Autodesk Inventor part; units mm, degrees
ref_plane "YZ Plane" through (0, 0, 0) normal (1, 0, 0) x (0, 1, 0)
ref_plane "XZ Plane" through (0, 0, 0) normal (0, 1, 0) x (-1, 0, 0)
ref_plane "XY Plane" through (0, 0, 0) normal (0, 0, 1) x (1, 0, 0)
sketch "Sketch3" plane through (0, 0, 0) normal (0, 1, 0) x (-1, 0, 0)
  line L0 (0, 0) -> (10, 0)
  line L1 (10, 0) -> (10, -10)
  line L2 (10, -10) -> (0, -10)
  line L3 (0, -10) -> (0, 0)
  dimension "d7" = 10
  dimension "d8" = 10
extrude "Extrusion1" add sketch "Sketch3" along normal blind 10
sketch "Sketch4" plane through (0, 0, 0) normal (1, 0, 0) x (0, 0, -1)
  line L0 (10, 0) -> (0, 0)
  line L1 (0, 0) -> (0, 10)
  line L2 (0, 0) -> (2.5, 0)
  line L3 (2.5, 0) -> (0, 2.3259)
  dimension "d11" = 2.5
extrude "Extrusion2" cut sketch "Sketch4" against normal blind 10
sketch "Sketch5" plane through (0, 0, -10) normal (1, 0, 0) x (0, 0, -1)
  line L0 (0, 0) -> (-7.5, 0)
  line L1 (0, 0) -> (0, 10)
  line L2 (-10, 10) -> (0, 10)
  line L3 (-10, 2.3259) -> (-10, 10)
  line L4 (-3.75, 0) -> (-3.75, 2.3259)
  line L5 (-3.75, 2.3259) -> (0, 4.4117)
  line L6 (0, 0) -> (-3.75, 0)
  line L7 (-1.5, 10) -> (-1.5, 6)
  line L8 (-1.5, 6) -> (-4.6791, 10)
  point P0 (-10, 0)
  dimension "d14" = 4
extrude "Extrusion3" cut sketch "Sketch5" against normal blind 10 contours L0 L4 L5 L1
sketch "Sketch6" plane through (0, 10, 0) normal (1, 0, 0) x (0, 0, -1)
  line L0 (0, 0) -> (10, 0)
  line L1 (6.25, -10) -> (2.5, -10)
  line L2 (8.75, 0) -> (8.75, -4.6256)
  line L3 (8.75, -4.6256) -> (5, 0)
  line L4 (5, 0) -> (8.75, 0)
  point P0 (0, -10)
extrude "Extrusion4" cut sketch "Sketch6" against normal blind 10
sketch "Sketch7" plane through (0, 2.3259, 0) normal (1, 0, 0) x (0, 0, -1)
  line L0 (0, 7.6741) -> (5, 7.6741)
  line L1 (0, 0) -> (0, 7.6741)
  line L2 (3.0747, 7.6741) -> (0, 7.6741)
  line L3 (0, 7.6741) -> (0, 2.0858)
  line L4 (0, 2.0858) -> (3.0747, 2.0858)
  line L5 (3.0747, 2.0858) -> (3.0747, 7.6741)
  point P0 (0, -2.3259)
extrude "Extrusion5" cut sketch "Sketch7" against normal blind 10
properties part number "136"
Build history of the part. All positions in model axes, mm. A direction names the side the tool comes from. Round coordinates to 2 decimals unless told otherwise and drop trailing zeros. Write each loop counter-clockwise with the first axis right and the second up, starting at its lowest first coordinate (ties: lowest second). Pieces come first, ordered by that corner, then holes.
1) Drill centre lines: probe 1 along Z at (x, y) = (-3, 7); probe 2 along Z at (x, y) = (-8.5, 9.25); probe 3 along Z at (x, y) = (-6.25, 4). Where is each one in solid material? Low to high.
2) 3-axis set-ups, long thin cutter, end or side, ignore diameter. For faces 1 (the flat face through (-5, 10, -4)), 2 (the flat face through (-5, 1, -6.25)), 3 (the flat face through (-5, 7, -3.075)): which of +Z, -Z, +X, -X, +Y, -Y reach the whole face in a straight line?
3) Mould opens along Z. For faces 4 (the flat face through (-5, 8, -8.75)), 5 (the flat face through (-5, 4.412, -2)), 6 (the flat face through (-4.93, 7.655, -6.901)), 7 (the flat face through (-4.93, 3.354, -8.099)) say: +Z half, -Z half, draft (parallel to the pull), parting line (faces both ways), or undercut.
4) Band-saw the part on C-C, the plane y = 5. List the corners of the cut face in (x, z).
5) Band-saw the part on A-A, the plane x = -1.5. List the corners of the cut face in (y, z), and give its area (3 significant figures).
6) Band-saw the part on D-D, the plane y = 6.5. List the corners of the cut face in (x, z).
7) Band-saw the part on B-B, the plane y = 9. List the corners of the cut face in (x, z), and give its area (3 significant figures).
8) Pin check, flat tips, straight feed: pin 1 (6 mm diameter, centred on x = -8.5, z = -7.5, fed in from -Y); pin 2 (2.5 mm diameter, centred on x = -2.5, y = 7, fed in from +Z); pin 3 (1 mm diameter, centred on x = -1.5, z = -7, fed in from -Y); pin 4 (0.7 mm diameter, centred on x = -6, y = 1.5, fed in from -Z). Stop position of each tip, or through.
Ans:
1. probe 1: z = -10 to -8.75, -7.43 to -3.07
1. probe 2: z = -10 to -8.75, -5.61 to -3.07
1. probe 3: z = -9.26 to 0
2. face 1: +Z, -Z, +X, -X, +Y
2. face 2: -Z, +X, -X, -Y
2. face 3: +Z, +X, -X, +Y
3. face 4: undercut
3. face 5: draft
3. face 6: undercut
3. face 7: -Z half
4. outline: (-10, -10) - (0, -10) - (0, -3.07) - (-10, -3.07) - close
5. outline: (0, -6.25) - (2.33, -6.25) - (4.41, -10) - (10, -10) - (10, -8.75) - (5.37, -8.75) - (10, -5) - (10, -3.07) - (4.41, -3.07) - (4.41, 0) - (2.33, 0) - (0, -2.5) - close
5. area: 58.6 mm2
6. outline: (-10, -10) - (0, -10) - (0, -8.75) - (-10, -8.75) - close; (-10, -7.84) - (0, -7.84) - (0, -3.07) - (-10, -3.07) - close
7. outline: (-10, -10) - (0, -10) - (0, -8.75) - (-10, -8.75) - close; (-10, -5.81) - (0, -5.81) - (0, -3.07) - (-10, -3.07) - close
7. area: 39.9 mm2
8. pin 1: stops at y = 0
8. pin 2: stops at z = -3.07
8. pin 3: stops at y = 2.46
8. pin 4: stops at z = -6.25
